Can you work these out from the model? Positions are in its coordinate system, mm. A direction names the side the tool comes from. Coordinates: 2 decimals unless noted, no trailing zeros. Write each loop counter-clockwise with the first axis right and the second up, starting at its lowest first coordinate (ties: lowest second). Pieces come first, ordered by that corner, then holes. Notation, with made-up numbers: (-21, 24) -> (0, 24) arc R26 cw to (0, 63) -> close; hole circle Ø2 at (43, -5.75). An arc over 180 degrees is marked (long way). Use one line per item in the form item = value.
Autodesk Inventor part; units mm, degrees
ref_plane "YZ Plane" through (0, 0, 0) normal (1, 0, 0) x (0, 1, 0)
ref_plane "XZ Plane" through (0, 0, 0) normal (0, 1, 0) x (-1, 0, 0)
ref_plane "XY Plane" through (0, 0, 0) normal (0, 0, 1) x (1, 0, 0)
sketch "Sketch1" plane through (0, 0, 0) normal (0, 0, 1) x (1, 0, 0)
  line L0 (-2.5718, -2.6632) -> (-7.5718, -2.6632)
  line L1 (-7.5718, -2.6632) -> (-7.5718, -60.8132)
  line L2 (-7.5718, -60.8132) -> (-2.5718, -60.8132)
  line L3 (-2.5718, -60.8132) -> (-2.5718, -2.6632)
  dimension "d1" = 58.15
  dimension "d2" = 5
revolve "Shoulder" add sketch "Sketch1" angle 360 about axis through (-2.5718, -60.8132, 0) along (0, 1, 0)
sketch "Sketch2" plane through (-2.5718, -2.6632, 0) normal (0, 1, 0) x (1, 0, 0)
  circle A0 centre (0, 0) radius 5
  circle A1 centre (0, 0) radius 4.76
  dimension "d3" = 9.52
extrude "Shoulder_neck" add sketch "Sketch2" along normal blind 1.85 contours A1
sketch "Sketch3" plane through (-2.5718, -0.8132, 0) normal (0, 1, 0) x (1, 0, 0)
  circle A0 centre (0, 0) radius 4.76
  circle A1 centre (0, 0) radius 8.1
  dimension "d6" = 16.2
extrude "Head" add sketch "Sketch3" along normal blind 7 contours A0 | A1
sketch "Sketch4" plane through (-2.5718, -60.8132, 0) normal (0, -1, 0) x (1, 0, 0)
  circle A0 centre (0, 0) radius 5
  circle A1 centre (0, 0) radius 3.09
  dimension "d9" = 6.18
extrude "Thread_neck" add sketch "Sketch4" along normal blind 2.6 contours A1
sketch "Sketch5" plane through (-2.5718, -63.4132, 0) normal (0, -1, 0) x (1, 0, 0)
  circle A0 centre (0, 0) radius 3.09
  circle A1 centre (0, 0) radius 4
  dimension "d12" = 8
extrude "Thread_shoulder" add sketch "Sketch5" along normal blind 10.4 contours A0 | A1
sketch "Sketch6" plane through (-2.5718, 6.1868, 0) normal (0, 1, 0) x (1, 0, 0)
  circle A0 centre (0, 0) radius 8.1
  circle A1 centre (0, 0) radius 2.5 construction
  line L0 (-2.5, 1.4434) -> (-2.5, -1.4434)
  line L1 (-2.5, -1.4434) -> (0, -2.8868)
  line L2 (0, -2.8868) -> (2.5, -1.4434)
  line L3 (2.5, -1.4434) -> (2.5, 1.4434)
  line L4 (2.5, 1.4434) -> (0, 2.8868)
  line L5 (0, 2.8868) -> (-2.5, 1.4434)
  dimension "d15" = 5
extrude "Hex" cut sketch "Sketch6" against normal blind 4.2 contours L5 L4 L3 L2 L1 L0
chamfer "Chamfer1" distance 0.24 angle 30 1 edges at (2.4282, -2.6632, 0) measured on face at (-7.3973, -2.6632, -0.7786)
fillet "Fillet1" radius 0.4 1 edges at (-7.3318, -0.8132, 0)
chamfer "Chamfer2" distance 0.5 angle 30 1 edges at (-10.6718, 6.1868, 0) measured on face at (5.4233, 3.8535, 1.2993)
chamfer "Chamfer3" distance 0.625 angle 30 1 edges at (-6.5718, -73.8132, 0) measured on face at (-1.8144, -73.8132, 1.0973)
fillet "Fillet2" radius 0.7 1 edges at (-5.6618, -60.8132, 0)
chamfer "Chamfer7" distance 0.91 angle 30 1 edges at (-6.5718, -63.4132, 0) measured on face at (1.0861, -63.4132, -0.3191)
thread "Thread"
equation "\"d1\" = Shoulder_length - Shoulder_neck_length"
equation "\"d2\" = 0.5 * Shoulder_diameter"
equation "\"d3\" = Shoulder_neck_dia"
equation "\"d4\" = Shoulder_neck_length"
equation "\"d6\" = Head_diameter"
equation "\"d7\" = Head_height"
equation "\"d9\" = Thread_neck_dia"
equation "\"d10\" = Thread_neck_length"
equation "\"d12\" = Thread_diameter"
equation "\"d13\" = Thread_length - Thread_neck_length"
equation "\"d15\" = Hex_size"
equation "\"d16\" = Hex_length"
equation "\"d18\" = -0.5 * Shoulder_neck_dia + 0.5 * Shoulder_diameter"
equation "\"d64\" = -0.5 * Shoulder_neck_dia + 0.5 * Shoulder_diameter"
equation "\"d21\" = 0.1 * Hex_size"
equation "\"d65\" = 0.1 * Hex_size"
equation "\"d23\" = 0.5 * Thread_pitch"
equation "\"d66\" = 0.5 * Thread_pitch"
equation "\"d25\" = Thread_neck_radius"
equation "\"d60\" = -0.5 * Thread_neck_dia + 0.5 * Thread_diameter"
equation "\"d67\" = -0.5 * Thread_neck_dia + 0.5 * Thread_diameter"
equation "\"Shoulder_length\" = 60"
equation "\"Shoulder_neck_dia\" = 9.52"
equation "\"Thread_diameter\" = 8"
equation "\"Thread_length\" = 13"
equation "\"Head_diameter\" = 16.2"
equation "\"Head_height\" = 7"
equation "\"Thread_neck_dia\" = 6.18"
equation "\"Hex_size\" = 5"
equation "\"Hex_length\" = 4.2"
equation "\"Thread_pitch\" = 1.25"
equation "\"Shoulder_neck_length\" = 1.85"
equation "\"Thread_neck_length\" = 2.6"
equation "\"Thread_neck_radius\" = 0.7"
properties part number "SCREW, SHOULDER, P, 12.9, 10X60" material "Steel, High Strength Low Alloy"
Q1. If I drill on line 1 (Y direction, x = -8.5, z = 2); line 2 (Z direction, x = 1.5, y = -41.5); line 3 (Y direction, x = -4.25, z = -0.75), over which ranges is the centre line in solid material (lowest first)? Write a range as from..to.
Return value:
line_1 = -0.81..6.19
line_2 = -2.9..2.9
line_3 = -73.81..1.99
Q2. Will these pins go through, and if not, where does the flat tip stop? pin 1 (1.4 mm diameter, centred on y = 4, z = -0.5, fed in from +X); pin 2 (2 mm diameter, centred on y = -65, z = -3.5, fed in from -X); pin 3 (6 mm diameter, centred on x = -5, y = -46.5, fed in from +Z); pin 4 (1.5 mm diameter, centred on y = -65, z = -2.5, fed in from +X).
Return value:
pin_1 = 5.53
pin_2 = -5.69
pin_3 = 5
pin_4 = 1.03
Q3. Thinking about a two-plate mould opening in Y: for faces 4 (the flat face through (1, 6.187, 0)), 5 (the flat face through (3, -0.813, 0)), 6 (the cylindrical face through (-6.349, -1.948, -2.896)), 7 (the cylindrical face through (-4.328, 2.391, -7.907)), which applies, released by +Y, released by -Y, zero draft, split by the parting line, or undercut?
Return value:
face_4 = released by +Y
face_5 = released by -Y
face_6 = undercut
face_7 = zero draft
Q4. Suppose I cut it at A-A (y = -45). Write out the boundary of the cut face in (x, z), then the cut area to 3 significant figures.
Return value:
outline = circle Ø10 at (-2.57, 0)
area = 78.5 mm2
Q5. For faces 1 (the flat face through (-1.339, 4.116, 2.175)), 2 (the cylindrical face through (-1.49, -32.21, 4.88)), 3 (the cylindrical face through (-0.9, -62.4, -2.6)), which set-ups out of +Z, -Z, +X, -X, +Y, -Y let a thin tool reach every point of the face, with its end or its side?
Return value:
face_1 = +Y
face_2 = -Y
face_3 = none
